Drawing for the job (mm, zero at the part's lowest x, y, z). Give positions to 0.01 mm unless a question says otherwise; leave off trailing zeros. Loops run counter-clockwise (first coordinate to the right, second up) from the corner with the lowest first, then second, coordinate; pieces in that order, holes last. Notation, with made-up numbers: M -6.5,19 L -2.5,19 A33 cw -2.5,48 Z; hole C 78.5,61 d8. An arc over 180 degrees is marked long. Use CSV: the item, a comma, the result in double quotes. Start each with the question number.
(1) Slice it at C-C on x = 38.1. List the corners of the cut face in (y, z).
(2) Flat gauge pin, fed straight in: P1, Ø8, axis at x = 19.5, y = 75, coming from the -Z side. Where does the tip first touch, or does it go through?
(3) Slice it at B-B on z = 22. List the corners of the cut face in (x, y), and give its area (3 significant figures).
(4) Wall check: line 1 along Z through (x, y) = (6.5, 60.5); line 2 along Y through (x, z) = (106, 15.5); line 3 along Y through (x, z) = (41, 28). Give the ranges that are in metal, low to high. Write a range as from..to.
(5) Slice it at A-A on y = 70. List the corners of the cut face in (x, z).
(6) Two-plate mould, pull along X, no slides. Class the marked faces 1 and 2: pulls with the +X half, pulls with the -X half, needs draft (parallel to the pull), parting line crosses it, or undercut.
(7) Slice it at D-D on y = 52. List the corners of the cut face in (x, z), and give its area (3 significant figures).
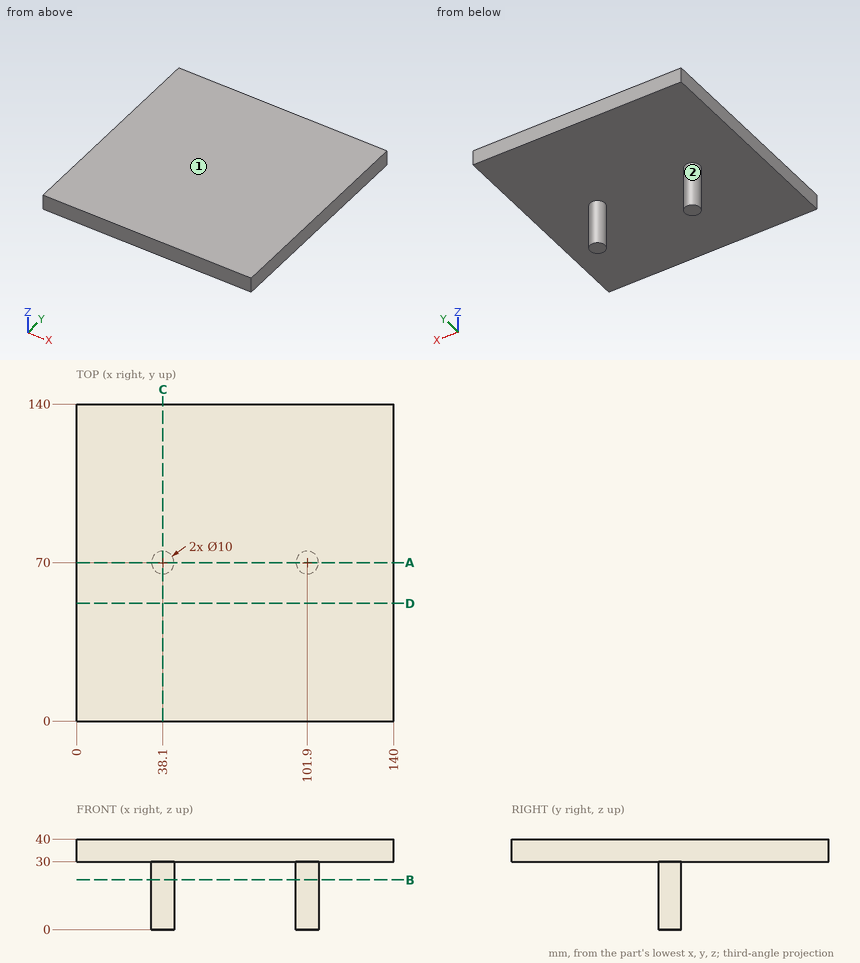
Reply:
1,outline,"M 0,30 L 65,30 L 65,0 L 75,0 L 75,30 L 140,30 L 140,40 L 0,40 Z"
2,P1,"stops at z = 30"
3,outline,"C 38.1,70 d10; C 101.9,70 d10"
3,area,"157 mm^2"
4,line 1,"z = 30..40"
4,line 2,"y = 67.14..72.86"
4,line 3,"y = 65.93..74.07"
5,outline,"M 0,30 L 33.1,30 L 33.1,0 L 43.1,0 L 43.1,30 L 96.9,30 L 96.9,0 L 106.9,0 L 106.9,30 L 140,30 L 140,40 L 0,40 Z"
6,face 1,"needs draft"
6,face 2,"undercut"
7,outline,"M 0,30 L 140,30 L 140,40 L 0,40 Z"
7,area,"1,400 mm^2"
